Model file for the job. Use its own axes, mm. A direction names the side the tool comes from. Give positions to 0.01 mm unless a question says otherwise; leave off trailing zeros. Order: outer loops, then holes, each group sorted by start corner. A loop starts at its lowest first (then second) coordinate and runs counter-clockwise, first axis right, second up. Notation, with made-up numbers: (-5.75, -32.5) - (6.25, -32.5) arc R27 ccw to (6.25, -15.5) - close; hole circle Ø9 at (-20, 29). An arc over 180 degrees is marked (long way). Use CSV: the item, a comma, the result in double quotes. Start each with the question number.
(1) Pull direction Y, two halves, no side cores. Call faces 4 (the flat face through (-2.5, -2.5, 7.5)), 5 (the cylindrical face through (-2.739, -2.826, 7.246)), 6 (the cylindrical face through (-5.158, -3.955, 3.451)): +Y half, -Y half, draft (parallel to the pull), parting line (faces both ways), or undercut.
(2) Band-saw the part on B-B, the plane x = 1.25. Give the cut face in (y, z), then the cut area to 3 significant figures.
(3) Band-saw the part on A-A, the plane z = 2.5. Give the cut face in (x, y), then the cut area to 3 significant figures.
(4) Tool access for faces 1 (the cylindrical face through (2.715, -2.849, 7.246)), 2 (the flat face through (2.5, 2.6, 7.5)), 3 (the flat face through (-0.82, -4.09, 3.55)): list every direction of +Z, -Z, +X, -X, +Y, -Y with a clear straight run to the whole face (end or side of a thin tool).
(5) Probe L1, parallel to X at y = -3, z = 4; L2, parallel to Y at x = -3, z = 5.5; L3, parallel to Y at x = -1, z = 5.5. List the from-to ranges inside material, lowest first.
(6) Band-saw the part on D-D, the plane y = 1. Give the cut face in (x, z).
(7) Drop flat-ended pins along their axis: pin 1 Ø4 at (x, z) = (-3.5, 3.5) entering from -Y; pin 2 Ø2 at (x, y) = (0.5, 1) entering from +Z. Give the stop position or say it passes through.
(8) Band-saw the part on C-C, the plane y = -3.5. Give the cut face in (x, z), then the cut area to 3 significant figures.
from build123d import *

# Parameters (mm, degrees)
F0_R     = 6.5
F0_R_2   = 2
F1_DEPTH = 7
F3_DEPTH = 25
F4_DEPTH = 0.5


with BuildPart() as f1:
    # F0 (on Top) → F1 (new body)
    with BuildSketch(Plane.XY):
        Circle(F0_R)
        Circle(F0_R_2, mode=Mode.SUBTRACT)
    extrude(amount=F1_DEPTH)

    # F2 (on face) → F3 (cut)
    with BuildSketch(Plane.XY.offset(7)):
        with BuildLine():
            ThreePointArc((-2.775807, -1.735036), (-3.273446, 0), (-2.775807, 1.735036))
            Line((-2.775807, 1.735036), (-5.223183, 0))
            Line((-5.223183, 0), (-2.775807, -1.735036))
        make_face()
        with BuildLine():
            Line((0, -5.365163), (1.623553, -2.842451))
            ThreePointArc((1.623553, -2.842451), (0, -3.273446), (-1.623553, -2.842451))
            Line((-1.623553, -2.842451), (0, -5.365163))
        make_face()
        with BuildLine():
            ThreePointArc((2.775807, 1.735036), (3.146578, 0.902496), (3.273446, 0))
            ThreePointArc((3.273446, 0), (3.146578, -0.902496), (2.775807, -1.735036))
            Line((2.775807, -1.735036), (5.223183, 0))
            Line((5.223183, 0), (2.775807, 1.735036))
        make_face()
        with BuildLine():
            ThreePointArc((-1.623553, 2.842451), (0, 3.273446), (1.623553, 2.842451))
            Line((1.623553, 2.842451), (0, 5.365163))
            Line((0, 5.365163), (-1.623553, 2.842451))
        make_face()
    extrude(amount=-F3_DEPTH, mode=Mode.SUBTRACT)

    # F2 (on face) → F4 (join)
    with BuildSketch(Plane.XY.offset(7)):
        with BuildLine():
            ThreePointArc((1.623553, 2.842451), (2.2683, 2.360142), (2.775807, 1.735036))
            ThreePointArc((2.775807, 1.735036), (2.780742, 2.893332), (1.623553, 2.842451))
        make_face()
        with BuildLine():
            ThreePointArc((-2.775807, 1.735036), (-2.2683, 2.360142), (-1.623553, 2.842451))
            ThreePointArc((-1.623553, 2.842451), (-2.780742, 2.893332), (-2.775807, 1.735036))
        make_face()
        with BuildLine():
            ThreePointArc((-2.775807, -1.735036), (-2.727321, -2.837748), (-1.623553, -2.842451))
            ThreePointArc((-1.623553, -2.842451), (-2.2683, -2.360142), (-2.775807, -1.735036))
        make_face()
        with BuildLine():
            ThreePointArc((1.623553, -2.842451), (2.727321, -2.837748), (2.775807, -1.735036))
            ThreePointArc((2.775807, -1.735036), (2.2683, -2.360142), (1.623553, -2.842451))
        make_face()
    extrude(amount=F4_DEPTH)


solid = f1.part
Answer block:
1,face 4,"draft"
1,face 5,"undercut"
1,face 6,"parting line"
2,outline,"(-6.38, 0) - (-3.42, 0) - (-3.42, 7) - (-6.38, 7) - close; (-3.03, 0) - (-1.56, 0) - (-1.56, 7) - (-3.03, 7) - close; (1.56, 0) - (3.03, 0) - (3.03, 7) - (1.56, 7) - close; (3.42, 0) - (6.38, 0) - (6.38, 7) - (3.42, 7) - close"
2,area,"61.9 mm2"
3,outline,"circle Ø13 at (0, 0); hole (-5.22, 0) - (-2.78, -1.74) arc R3.27 cw to (-2.78, 1.74) - close; hole circle Ø4 at (0, 0); hole (-1.62, -2.84) - (0, -5.37) - (1.62, -2.84) arc R3.27 cw to start; hole (-1.62, 2.84) arc R3.27 cw to (1.62, 2.84) - (0, 5.37) - close; hole (2.78, -1.74) - (5.22, 0) - (2.78, 1.74) arc R3.27 cw to (3.27, 0) arc R3.27 cw to start"
3,area,"108 mm2"
4,face 1,"+Z"
4,face 2,"+Z, +X, -X, +Y, -Y"
4,face 3,"+Z, -Z"
5,L1,"x = -5.77 to -1.52, -1.31 to 1.31, 1.52 to 5.77"
5,L2,"y = -5.77 to -1.58, -1.31 to 1.31, 1.58 to 5.77"
5,L3,"y = -6.42 to -3.81, -3.12 to -1.73, 1.73 to 3.12, 3.81 to 6.42"
6,outline,"(-6.42, 0) - (-3.81, 0) - (-3.81, 7) - (-6.42, 7) - close; (-3.12, 0) - (-1.73, 0) - (-1.73, 7) - (-3.12, 7) - close; (1.73, 0) - (3.12, 0) - (3.12, 7) - (1.73, 7) - close; (3.81, 0) - (6.42, 0) - (6.42, 7) - (3.81, 7) - close"
7,pin 1,"stops at y = -6.32"
7,pin 2,"stops at z = 7"
8,outline,"(-5.48, 0) - (-1.2, 0) - (-1.2, 7) - (-5.48, 7) - close; (1.2, 0) - (5.48, 0) - (5.48, 7) - (1.2, 7) - close"
8,area,"59.9 mm2"
